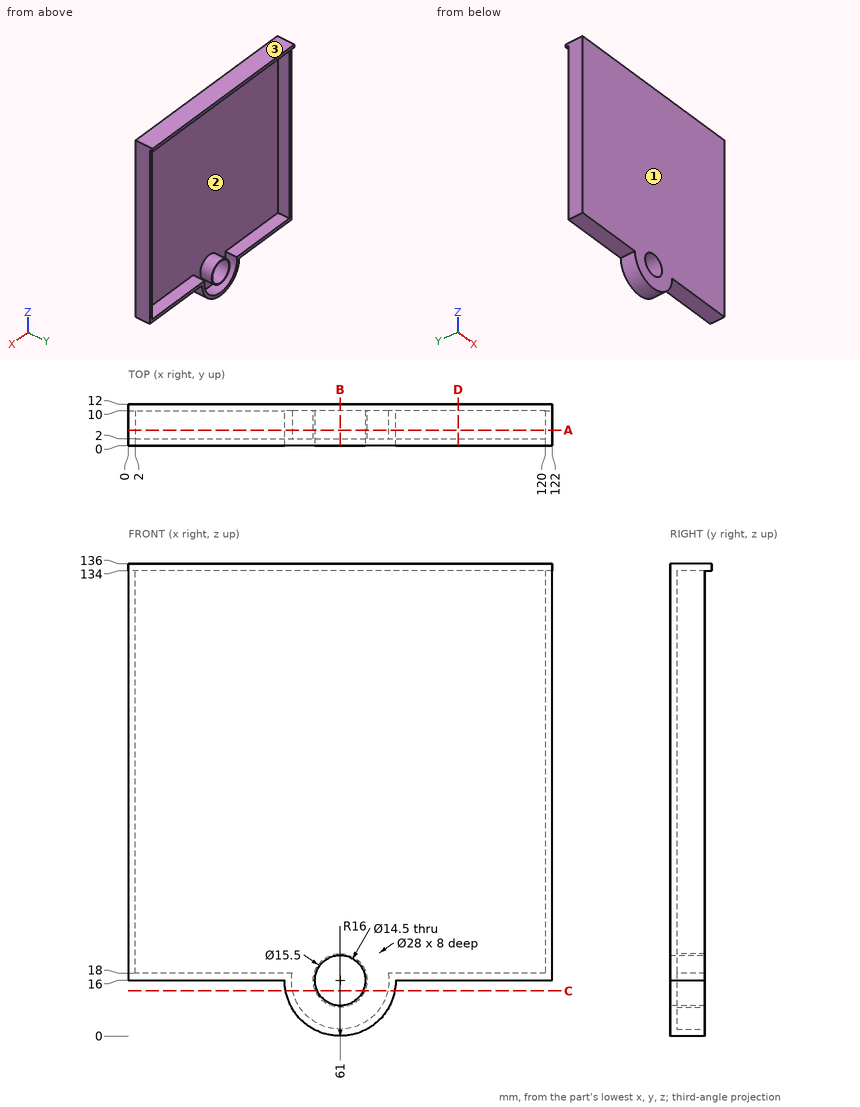
Study the drawing (mm; zero at the part's minimum x, y, z) and answer. Give positions to 0.01 mm unless a question says otherwise; leave off trailing zeros. Loops run counter-clockwise (first coordinate to the right, second up) from the corner with the lowest first, then second, coordinate; pieces in that order, holes last. Notation, with made-up numbers: (-32.5, 11.5) -> (-1.5, 11.5) arc R11 cw to (-1.5, 17.5) -> close; hole circle Ø4 at (-28.75, 2). An arc over 180 degrees is marked (long way). Use a Markdown table: item, result. Add a question column.
1) The part is cut by section B-B, the plane x = 61. Determine the outline of the cut face in (y, z).
2) For a pull along Z with two mould halves and no side action, classify the marked faces 1, 2 and 3 as +Z half, -Z half, draft (parallel to the pull), parting line (faces both ways), or undercut.
3) The part is cut by section D-D, the plane x = 95. Determine the outline of the cut face in (y, z), plus the area to 3 significant figures.
4) Consider line 1 along Z through (x, y) = (36.5, 7); line 2 along Z through (x, y) = (57.5, 9.75); line 3 along X through (y, z) = (2.25, 36.5). Determine where each line is inside the solid, lowest interval first.
5) The part is cut by section A-A, the plane y = 4.5. Determine the outline of the cut face in (x, z), plus the area to 3 significant figures.
6) Each of these flat-tipped pins is pushed along its axis until it touches: P1, Ø23, axis at x = 61, z = 16, coming from the +Y side; P2, Ø5, axis at x = 13.5, y = 7, coming from the -Z side; P3, Ø12, axis at x = 107.5, z = 100, coming from the +Y side; P4, Ø25, axis at x = 61, z = 16, coming from the -Y side. Where does it stop, or does it pass through?
7) The part is cut by section C-C, the plane z = 13. Determine the outline of the cut face in (x, y).
Reported:
| question | item | result |
|---|---|---|
| 1 | outline | (0, 0) -> (10, 0) -> (10, 2) -> (2, 2) -> (2, 8.25) -> (10, 8.25) -> (10, 8.75) -> (0, 8.75) -> close; (0, 23.25) -> (10, 23.25) -> (10, 23.75) -> (2, 23.75) -> (2, 134) -> (12, 134) -> (12, 136) -> (0, 136) -> close |
| 2 | face 1 | draft |
| 2 | face 2 | undercut |
| 2 | face 3 | +Z half |
| 3 | outline | (0, 16) -> (10, 16) -> (10, 18) -> (2, 18) -> (2, 134) -> (12, 134) -> (12, 136) -> (0, 136) -> close |
| 3 | area | 276 mm^2 |
| 4 | line 1 | z = 16 to 18, 134 to 136 |
| 4 | line 2 | z = 0.39 to 2.44, 9.09 to 9.65, 22.35 to 22.91, 134 to 136 |
| 4 | line 3 | x = 0 to 2, 120 to 122 |
| 5 | outline | (0, 16) -> (45, 16) arc R16 ccw to (77, 16) -> (122, 16) -> (122, 136) -> (0, 136) -> close; circle Ø15.5 at (61, 16); hole (2, 18) -> (47.14, 18) arc R14 ccw (long way) to (74.86, 18) -> (120, 18) -> (120, 134) -> (2, 134) -> close; hole circle Ø14.5 at (61, 16) |
| 5 | area | 1,010 mm^2 |
| 6 | P1 | stops at y = 10 |
| 6 | P2 | stops at z = 16 |
| 6 | P3 | stops at y = 2 |
| 6 | P4 | stops at y = 0 |
| 7 | outline | (45.28, 0) -> (54.4, 0) -> (54.4, 10) -> (53.85, 10) -> (53.85, 2) -> (47.33, 2) -> (47.33, 10) -> (45.28, 10) -> close; (67.6, 0) -> (76.72, 0) -> (76.72, 10) -> (74.67, 10) -> (74.67, 2) -> (68.15, 2) -> (68.15, 10) -> (67.6, 10) -> close |
